Input: part model. Units: mm. Frame: model coordinates. Face numbers are marked on the shaded views. A direction names the side the tool comes from. Coordinates: 2 decimals unless noted, no trailing zeros. Write each loop counter-clockwise with the first axis right and the second up, starting at its lowest first coordinate (ties: lowest second). Pieces come first, ordered by that corner, then holes. Notation, with made-up numbers: M -40,9.5 L -36,9.5 A19 cw -36,44.5 Z; hole C 18,46.5 d8. An arc over 180 degrees is marked long. Use one line per item in the form item = value.
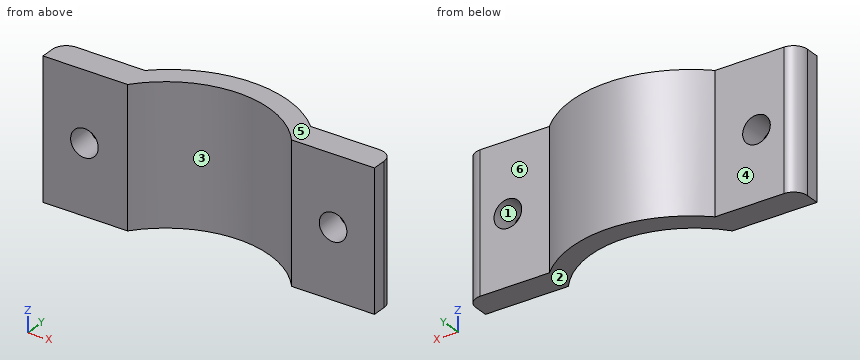
from build123d import *

# Parameters (mm, degrees)
BOSS_EXTRUDE1_DEPTH = 10
SKETCH3_R           = 1
CUT_EXTRUDE1_DEPTH  = 10
FILLET1_R           = 1


with BuildPart() as part:
    # Sketch2 → Boss-Extrude1 (new body)
    with BuildSketch(Plane.XY):
        with BuildLine():
            Line((-19.540356597, 0), (-19.540356597, -2))
            Line((-19.540356597, -2), (-13.418721915, -2))
            ThreePointArc((-13.418721915, -2), (-7.479539256, 0.9), (-1.540356597, -2))
            Line((-1.540356597, -2), (4.459643403, -2))
            Line((4.459643403, -2), (4.459643403, 0))
            Line((4.459643403, 0), (-1.540356597, 0))
            ThreePointArc((-1.540356597, 0), (-7.540356597, 2.439966221), (-13.540356597, 0))
            Line((-13.540356597, 0), (-19.540356597, 0))
        make_face()
    extrude(amount=BOSS_EXTRUDE1_DEPTH)

    # Sketch3 → Cut-Extrude1 (cut)
    with BuildSketch(Plane(origin=(0, 0, 0), x_dir=(1, 0, 0), z_dir=(0, 1, 0))):
        with Locations(Location((-16.540356597, -5, 0), (0, 0, 270))):
            Circle(SKETCH3_R)
        with Locations(Location((1.459643403, -5, 0), (0, 0, 270))):
            Circle(SKETCH3_R)
    extrude(amount=-CUT_EXTRUDE1_DEPTH, mode=Mode.SUBTRACT)

    # Fillet1
    fillet1_edges = [part.edges().sort_by_distance(p)[0] for p in [
        (4.459643403, 0, 5),
        (-19.540356597, 0, 5),
    ]]
    fillet(fillet1_edges, radius=FILLET1_R)


solid = part.part
(1) Pull-direction query (Z, two-part tool) for the marked faces 1, 2 and 3; classes: pulls with the +Z half, pulls with the -Z half, needs draft (parallel to the pull), parting line crosses it, or undercut.
Computed:
face_1 = undercut
face_2 = pulls with the -Z half
face_3 = needs draft
(2) Section query A-A on z = 5. Return the cut outline in (x, y).
Computed:
outline = M -19.54,-2 L -17.54,-2 L -17.54,0 L -18.54,0 A1 ccw -19.54,-1 Z; M -15.54,-2 L -13.42,-2 A7.53 cw -1.54,-2 L 0.46,-2 L 0.46,0 L -1.54,0 A8.6 ccw -13.54,0 L -15.54,0 Z; M 2.46,-2 L 4.46,-2 L 4.46,-1 A1 ccw 3.46,0 L 2.46,0 Z
(3) Set-up query: the marked faces 4, 5 and 6. Return all of +Z, -Z, +X, -X, +Y, -Y with unobstructed straight access to the full face (end or side cutting, diameter ignored); none if empty.
Computed:
face_4 = +Z, -Z, -X, +Y
face_5 = +Z, +X, -X, +Y, -Y
face_6 = +Z, -Z, +X, +Y
(4) Line query: probe 1 along X at (y, z) = (-0.9, 5); probe 2 along X at (y, z) = (-1.25, 5); probe 3 along Y at (x, z) = (3.25, 5.5). Output: solid intervals per line, ascending.
Computed:
probe_1 = -19.54 to -17.54, -15.54 to -12.37, -2.59 to 0.46, 2.46 to 4.45
probe_2 = -19.54 to -17.54, -15.54 to -12.75, -2.21 to 0.46, 2.46 to 4.46
probe_3 = -2 to 0
(5) First-contact query: pin 1 Ø2.5 at (x, z) = (-16.54, 5) entering from +Y; pin 2 Ø4 at (x, z) = (-6, 4) entering from -Y. Flat tips, straight axial feed; report the tip coordinate or a pass-through.
Computed:
pin_1 = 0
pin_2 = 0.05
(6) Section query D-D on x = -10.5. Return the cut outline in (y, z), plus the area to 3 significant figures.
Computed:
outline = M 0.27,0 L 1.91,0 L 1.91,10 L 0.27,10 Z
area = 16.5 mm^2
(7) Section query B-B on x = -16.25. Return the cut outline in (y, z).
Computed:
outline = M -2,0 L 0,0 L 0,4.04 L -2,4.04 Z; M -2,5.96 L 0,5.96 L 0,10 L -2,10 Z
(8) Section query C-C on z = 8.75. Return the cut outline in (x, y).
Computed:
outline = M -19.54,-2 L -13.42,-2 A7.53 cw -1.54,-2 L 4.46,-2 L 4.46,-1 A1 ccw 3.46,0 L -1.54,0 A8.6 ccw -13.54,0 L -18.54,0 A1 ccw -19.54,-1 Z
